Can you work these out from the model? Positions are in its coordinate system, mm. A direction names the side the tool comes from. Give positions to 0.01 mm unless a question says otherwise; leave off trailing zeros. Order: outer loops, then holes, each group sorted by start corner. A loop starts at its lowest first (then second) coordinate and runs counter-clockwise, first axis right, second up. Notation, with made-up numbers: M 31.25,62.5 L 84.25,62.5 A18 ccw 84.25,93.5 Z; hole C 75,-32 d2. An arc over 180 degrees is marked long. Use a Markdown table: item, result. Add a question column.
from build123d import *

# Parameters (mm, degrees)
F0_R     = 1.75
F1_DEPTH = 5


with BuildPart() as f1:
    # F0 (on Top) → F1 (new body)
    with BuildSketch(Plane.XY):
        with BuildLine():
            Line((-7.5, 13.5), (-7.5, -13.5))
            Line((-7.5, -13.5), (7.5, -13.5))
            Line((7.5, -13.5), (7.5, 13.5))
            Line((7.5, 13.5), (14.696938, 13.5))
            ThreePointArc((14.696938, 13.5), (0, 25.5), (-14.696938, 13.5))
            Line((-14.696938, 13.5), (-7.5, 13.5))
        make_face()
        with Locations((0, -9.3)):
            Circle(F0_R, mode=Mode.SUBTRACT)
        with Locations((0, 8)):
            Circle(F0_R, mode=Mode.SUBTRACT)
    extrude(amount=F1_DEPTH)


solid = f1.part
1. If we section it at D-D, the plane y = 9: List the corners of the cut face in (x, z) for me.
2. If we section it at A-A, the plane x = 0: List the corners of the cut face in (y, z) for me, then the cut area to 3 significant figures.
3. Will these pins go through, and if not, where does the flat tip stop? pin 1 (2.5 mm diameter, centred on x = 12.5, z = 1.5, fed in from -Y); pin 2 (1.5 mm diameter, centred on x = 6, z = 2.5, fed in from +Y); pin 3 (1.5 mm diameter, centred on y = -4.5, z = 3.5, fed in from -X); pin 4 (4 mm diameter, centred on x = -11, y = 4, fed in from -Z).
4. If we section it at B-B, the plane y = -9.3: List the corners of the cut face in (x, z) for me.
5. We'd pull the mould along Y, two halves only. Please class faces 1 (the face through (7.5, 0, 2)), 2 (the face through (11, 13.5, 2)), 3 (the face through (0.288, 25.497, 2.465)), 4 (the face through (-0.228, 9.735, 2.465)): +Y half, -Y half, draft (parallel to the pull), parting line (faces both ways), or undercut.
6. On a 3-axis mill with a long thin cutter (end or side, diameter ignored), from which of +Z, -Z, +X, -X, +Y, -Y can I reach the whole of each face in a straight line? I mean faces 5 (the face through (-7.5, 0, 2)), 6 (the face through (0, 11, 5)). Say none if no direction works.
7. I need wall thicknesses on L1, parallel to X at y = -6, z = 3.2; L2, parallel to Y at x = 0.5, z = 1.6; L3, parallel to X at y = 15, z = 4.1. Which ranges of each line are inside material? Lowest first, please. Write a range as [from, to].
8. If we section it at C-C, the plane z = 1.7: List the corners of the cut face in (x, y) for me.
Geometry results:
| question | item | result |
|---|---|---|
| 1 | outline | M -7.5,0 L -1.44,0 L -1.44,5 L -7.5,5 Z; M 1.44,0 L 7.5,0 L 7.5,5 L 1.44,5 Z |
| 2 | outline | M -13.5,0 L -11.05,0 L -11.05,5 L -13.5,5 Z; M -7.55,0 L 6.25,0 L 6.25,5 L -7.55,5 Z; M 9.75,0 L 25.5,0 L 25.5,5 L 9.75,5 Z |
| 2 | area | 160 mm^2 |
| 3 | pin 1 | stops at y = 13.5 |
| 3 | pin 2 | stops at y = 24.55 |
| 3 | pin 3 | stops at x = -7.5 |
| 3 | pin 4 | passes through |
| 4 | outline | M -7.5,0 L -1.75,0 L -1.75,5 L -7.5,5 Z; M 1.75,0 L 7.5,0 L 7.5,5 L 1.75,5 Z |
| 5 | face 1 | draft |
| 5 | face 2 | -Y half |
| 5 | face 3 | +Y half |
| 5 | face 4 | undercut |
| 6 | face 5 | +Z, -Z, -X, -Y |
| 6 | face 6 | +Z, +X, -X, +Y, -Y |
| 7 | L1 | x = [-7.5, 7.5] |
| 7 | L2 | y = [-13.5, -10.98], [-7.62, 6.32], [9.68, 25.49] |
| 7 | L3 | x = [-14.31, 14.31] |
| 8 | outline | M -14.7,13.5 L -7.5,13.5 L -7.5,-13.5 L 7.5,-13.5 L 7.5,13.5 L 14.7,13.5 A15 ccw Z; hole C 0,-9.3 d3.5; hole C 0,8 d3.5 |
